Source: three-view drawing plus pictorial views. Frame: mm from the lowest corner of the part. Round coordinates to 2 decimals unless told otherwise and drop trailing zeros. Write each loop counter-clockwise with the first axis right and the second up, starting at its lowest first coordinate (ties: lowest second). Pieces come first, ordered by that corner, then holes. Notation, with made-up numbers: M 9,21 L 17,21 A19 ccw 17,43 Z; hole C 32.25,78.5 d8. An arc over 180 degrees is marked long. Answer in a Markdown table with one row per item.
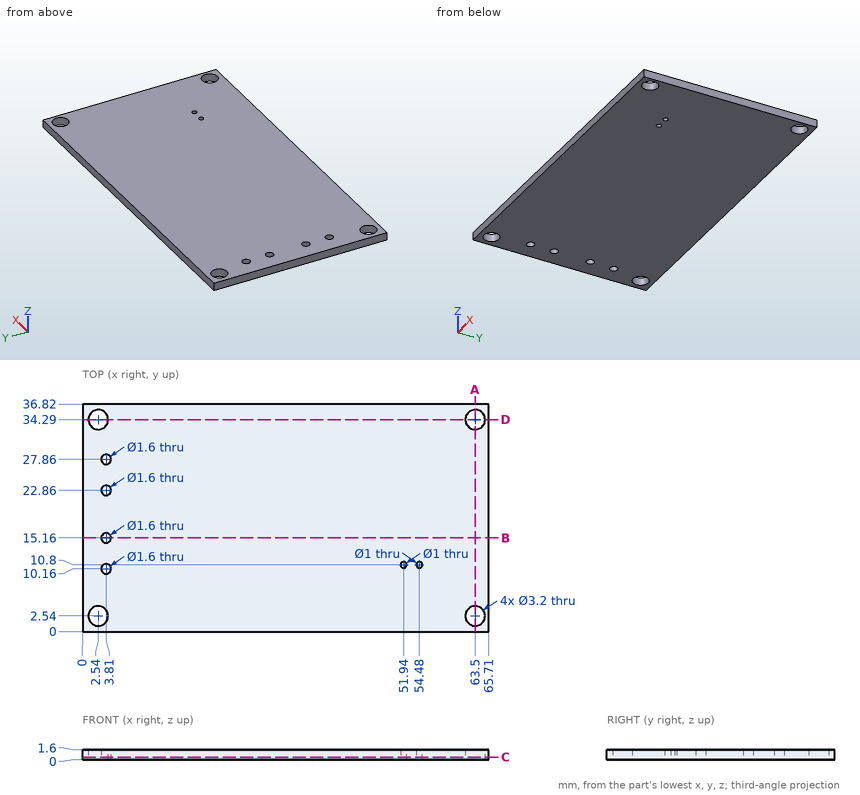
Q1. Material intervals for probe 1 along Y at (x, z) = (63.5, 0.3); probe 2 along Y at (x, z) = (51.94, 1.2); probe 3 along X at (y, z) = (35.5, 1.25), sorted ascending.
Solutions:
| item | result |
|---|---|
| probe 1 | y = 0 to 0.94, 4.14 to 32.69, 35.89 to 36.82 |
| probe 2 | y = 0 to 10.3, 11.3 to 36.82 |
| probe 3 | x = 0 to 1.49, 3.59 to 62.45, 64.55 to 65.71 |
Q2. Section C-C (z = 0.4). State how many separate pieces and enclosed holes the cut face has, and give its area (3 significant figures).
Solutions:
| item | result |
|---|---|
| separate pieces | 1 |
| enclosed holes | 10 |
| area | 2,380 mm2 |
Q3. Section A-A (x = 63.5). Return loops of the section in (y, z).
Solutions:
| item | result |
|---|---|
| outline | M 0,0 L 0.94,0 L 0.94,1.6 L 0,1.6 Z; M 4.14,0 L 32.69,0 L 32.69,1.6 L 4.14,1.6 Z; M 35.89,0 L 36.82,0 L 36.82,1.6 L 35.89,1.6 Z |
Q4. Section B-B (y = 15.16). Return loops of the section in (x, z), and give its area (3 significant figures).
Solutions:
| item | result |
|---|---|
| outline | M 0,0 L 3.01,0 L 3.01,1.6 L 0,1.6 Z; M 4.61,0 L 65.71,0 L 65.71,1.6 L 4.61,1.6 Z |
| area | 103 mm2 |
Q5. Section D-D (y = 34.29). Return loops of the section in (x, z).
Solutions:
| item | result |
|---|---|
| outline | M 0,0 L 0.94,0 L 0.94,1.6 L 0,1.6 Z; M 4.14,0 L 61.9,0 L 61.9,1.6 L 4.14,1.6 Z; M 65.1,0 L 65.71,0 L 65.71,1.6 L 65.1,1.6 Z |
